Source: CAD feature listing. Evaluate the final solid. Frame: model axes, mm. Face numbers are marked on the shaded views. A direction names the side the tool comes from. Round coordinates to 2 decimals unless told otherwise and drop trailing zeros. Write each loop counter-clockwise with the first axis right and the second up, starting at its lowest first coordinate (ties: lowest second). Pieces come first, ordered by that corner, then holes. Notation, with made-up numbers: (67.5, -15) - (114.5, -15) arc R21 ccw to (114.5, -8) - close; hole circle Ø5 at (51, 59.25). An arc over 180 degrees is marked (long way). Write item = value, one per line. Start each with the question number.
```python
from build123d import *

# Parameters (mm, degrees)
SKETCH1_W           = 75
SKETCH1_H           = 50
SKETCH1_R           = 7.5
SKETCH1_R_2         = 2.5
BOSS_EXTRUDE1_DEPTH = 50
SKETCH2_W           = 10
SKETCH2_H           = 20
CUT_EXTRUDE1_DEPTH  = 104.07764064


with BuildPart() as part:
    # Sketch1 → Boss-Extrude1 (new body)
    with BuildSketch(Plane.XY):
        with Locations((37.5, 25)):
            Rectangle(SKETCH1_W, SKETCH1_H)
        with Locations((20, 25)):
            Circle(SKETCH1_R, mode=Mode.SUBTRACT)
        with Locations((62, 25)):
            Circle(SKETCH1_R_2, mode=Mode.SUBTRACT)
    extrude(amount=BOSS_EXTRUDE1_DEPTH)

    # Sketch2 → Cut-Extrude1 (cut, through all)
    with BuildSketch(Plane(origin=(0, 50, 0), x_dir=(1, 0, 0), z_dir=(0, 1, 0))):
        with Locations((37.5, -20)):
            Rectangle(SKETCH2_W, SKETCH2_H)
    extrude(amount=-CUT_EXTRUDE1_DEPTH, mode=Mode.SUBTRACT)


solid = part.part
```
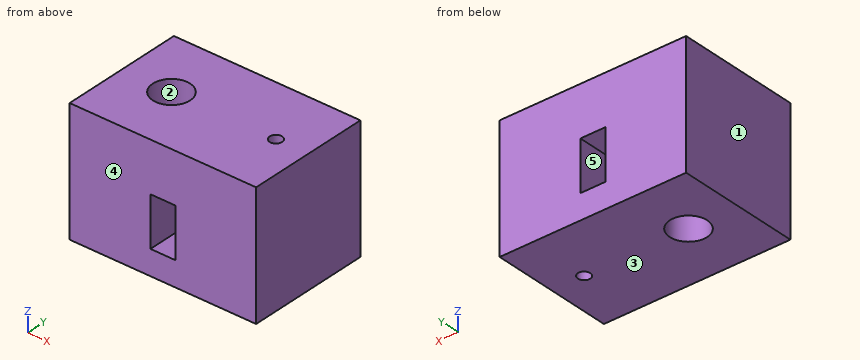
(1) Section B-B (x = 20). Return the cut outline in (y, z), plus the area to 3 significant figures.
(2) Reachability of the marked faces 4 and 5 from +Z, -Z, +X, -X, +Y, -Y: full face, straight path, thin tool, end or side. Return the list, or none.
(3) Ray query, L1, parallel to X at y = 12.5, z = 28; L2, parallel to Y at x = 20, z = 35; L3, parallel to Z at x = 36, y = 10. Return the intervals inside material, ascending. Write a range as from..to.
(4) Pull-direction query (X, two-part tool) for the marked faces 1, 2 and 3; classes: +X half, -X half, draft (parallel to the pull), parting line (faces both ways), or undercut.
(5) Section C-C (z = 8). Return the cut outline in (x, y), plus the area to 3 significant figures.
(6) Section D-D (y = 6.5). Return the cut outline in (x, z).
(7) Contact query for a flat-ended pin moving along its axis: P1, Ø1.5, axis at y = 31.5, z = 17.5, coming from the -X side. Output: stop coordinate, or through.
(8) Section A-A (y = 25). Return the cut outline in (x, z).
Solution:
q1.outline = (0, 0) - (17.5, 0) - (17.5, 50) - (0, 50) - close; (32.5, 0) - (50, 0) - (50, 50) - (32.5, 50) - close
q1.area = 1,750 mm^2
q2.face_4 = +Z, -Z, +X, -X, -Y
q2.face_5 = +Y, -Y
q3.L1 = 0..32.5, 42.5..75
q3.L2 = 0..17.5, 32.5..50
q3.L3 = 0..10, 30..50
q4.face_1 = -X half
q4.face_2 = undercut
q4.face_3 = draft
q5.outline = (0, 0) - (75, 0) - (75, 50) - (0, 50) - close; hole circle Ø15 at (20, 25); hole circle Ø5 at (62, 25)
q5.area = 3,550 mm^2
q6.outline = (0, 0) - (75, 0) - (75, 50) - (0, 50) - close; hole (32.5, 10) - (42.5, 10) - (42.5, 30) - (32.5, 30) - close
q7.P1 = 0
q8.outline = (0, 0) - (12.5, 0) - (12.5, 50) - (0, 50) - close; (27.5, 0) - (59.5, 0) - (59.5, 50) - (27.5, 50) - close; (64.5, 0) - (75, 0) - (75, 50) - (64.5, 50) - close; hole (32.5, 10) - (42.5, 10) - (42.5, 30) - (32.5, 30) - close
